from build123d import *

# Parameters (mm, degrees)
BOSS_EXTRU_1_DEPTH      = 10
ESQUISSE2_W             = 18.2
ESQUISSE2_H             = 8.4
ENL_V_MAT_EXTRU_1_DEPTH = 3
ESQUISSE3_R             = 1.6
ENL_V_MAT_EXTRU_2_DEPTH = 19.028865744
ESQUISSE4_R             = 3
ENL_V_MAT_EXTRU_3_DEPTH = 3
CONG_1_R                = 1.5


with BuildPart() as part:
    # Esquisse1 → Boss.-Extru.1 (new body)
    with BuildSketch(Plane(origin=(0, 0, 0), x_dir=(1, 0, 0), z_dir=(0, 1, 0))):
        Polygon((2.4, 0), (11, 0), (11, -9), (-11, -9), (-11, 0), (-2.4, 0), (-2.4, 1.2), (2.4, 1.2), align=None)
    extrude(amount=BOSS_EXTRU_1_DEPTH)

    # Esquisse2 → Enlèv. mat.-Extru.1 (cut)
    with BuildSketch(Plane(origin=(0, 10, 0), x_dir=(1, 0, 0), z_dir=(0, 1, 0))):
        with Locations((0, -3)):
            Rectangle(ESQUISSE2_W, ESQUISSE2_H)
    extrude(amount=-ENL_V_MAT_EXTRU_1_DEPTH, mode=Mode.SUBTRACT)

    # Esquisse3 → Enlèv. mat.-Extru.2 (cut, through all)
    with BuildSketch(Plane(origin=(0, 0, -1.2), x_dir=(-1, 0, 0), z_dir=(0, 0, -1))):
        with Locations((0, 3.5)):
            Circle(ESQUISSE3_R)
    extrude(amount=-ENL_V_MAT_EXTRU_2_DEPTH, mode=Mode.SUBTRACT)

    # Esquisse4 → Enlèv. mat.-Extru.3 (cut)
    with BuildSketch(Plane.XY.offset(9)):
        with Locations((0, 3.5)):
            Circle(ESQUISSE4_R)
    extrude(amount=-ENL_V_MAT_EXTRU_3_DEPTH, mode=Mode.SUBTRACT)

    # Congé1
    # the kernel refuses this fillet: 1.5 mm, written as the material it takes off along each edge
    with BuildSketch(Plane(origin=(9.5, 8.5, 7.5), x_dir=(0, 1, 0), z_dir=(1, 0, 0))) as cong_1_piece_1_section:
        Polygon((0, 0), (CONG_1_R, 0), (CONG_1_R, CONG_1_R), (0, CONG_1_R), align=None)
    cong_1_piece_1 = extrude(amount=CONG_1_R, mode=Mode.PRIVATE)
    cong_1_piece_1 = cong_1_piece_1 - Plane(origin=(9.5, 8.5, 7.5), x_dir=(0, -0.7071067811865475, -0.7071067811865475), z_dir=(1, 0, 0)) * Sphere(CONG_1_R, mode=Mode.PRIVATE)
    add(cong_1_piece_1, mode=Mode.SUBTRACT)
    with BuildSketch(Plane(origin=(9.5, 1.5, 7.5), x_dir=(1, 0, 0), z_dir=(0, -1, 0))) as cong_1_piece_2_section:
        Polygon((0, 0), (CONG_1_R, 0), (CONG_1_R, CONG_1_R), (0, CONG_1_R), align=None)
    cong_1_piece_2 = extrude(amount=CONG_1_R, mode=Mode.PRIVATE)
    cong_1_piece_2 = cong_1_piece_2 - Plane(origin=(9.5, 1.5, 7.5), x_dir=(-0.7071067811865476, 0, -0.7071067811865475), z_dir=(0, -1, 0)) * Sphere(CONG_1_R, mode=Mode.PRIVATE)
    add(cong_1_piece_2, mode=Mode.SUBTRACT)
    with BuildSketch(Plane(origin=(-9.5, 1.5, 7.5), x_dir=(0, -1, 0), z_dir=(-1, 0, 0))) as cong_1_piece_3_section:
        Polygon((0, 0), (CONG_1_R, 0), (CONG_1_R, CONG_1_R), (0, CONG_1_R), align=None)
    cong_1_piece_3 = extrude(amount=CONG_1_R, mode=Mode.PRIVATE)
    cong_1_piece_3 = cong_1_piece_3 - Plane(origin=(-9.5, 1.5, 7.5), x_dir=(0, 0.7071067811865475, -0.7071067811865475), z_dir=(-1, 0, 0)) * Sphere(CONG_1_R, mode=Mode.PRIVATE)
    add(cong_1_piece_3, mode=Mode.SUBTRACT)
    with BuildSketch(Plane(origin=(-9.5, 8.5, 7.5), x_dir=(0, 1, 0), z_dir=(-1, 0, 0))) as cong_1_piece_4_section:
        Polygon((0, 0), (CONG_1_R, 0), (CONG_1_R, -CONG_1_R), (0, -CONG_1_R), align=None)
    cong_1_piece_4 = extrude(amount=CONG_1_R, mode=Mode.PRIVATE)
    cong_1_piece_4 = cong_1_piece_4 - Plane(origin=(-9.5, 8.5, 7.5), x_dir=(0, -0.7071067811865475, -0.7071067811865475), z_dir=(-1, 0, 0)) * Sphere(CONG_1_R, mode=Mode.PRIVATE)
    add(cong_1_piece_4, mode=Mode.SUBTRACT)
    with BuildSketch(Plane(origin=(11, 10, -3.75), x_dir=(0, -1, 0), z_dir=(0, 0, 1)), Plane(origin=(-11, 0, 7.5), x_dir=(1, 0, 0), z_dir=(0, 0, -1)), Plane(origin=(11, 0, -3.75), x_dir=(-1, 0, 0), z_dir=(0, 0, 1))) as cong_1_piece_5:
        with BuildLine():
            CenterArc((CONG_1_R, -CONG_1_R), CONG_1_R, 90, 90)
            Line((0, -CONG_1_R), (0, 0))
            Line((0, 0), (CONG_1_R, 0))
        make_face()
    extrude(amount=11.25, mode=Mode.SUBTRACT)
    with BuildSketch(Plane(origin=(9.5, 0, 9), x_dir=(0, 0, -1), z_dir=(-1, 0, 0))) as cong_1_piece_6:
        with BuildLine():
            CenterArc((CONG_1_R, -CONG_1_R), CONG_1_R, 90, 90)
            Line((0, -CONG_1_R), (0, 0))
            Line((0, 0), (CONG_1_R, 0))
        make_face()
    extrude(amount=19, mode=Mode.SUBTRACT)
    with BuildSketch(Plane(origin=(-11, -3.75, 0), x_dir=(0, 0, 1), z_dir=(0, 1, 0)), Plane(origin=(11, -3.75, 0), x_dir=(-1, 0, 0), z_dir=(0, 1, 0))) as cong_1_piece_7:
        with BuildLine():
            CenterArc((CONG_1_R, CONG_1_R), CONG_1_R, 180, 90)
            Line((0, CONG_1_R), (0, 0))
            Line((0, 0), (CONG_1_R, 0))
        make_face()
    extrude(amount=17.5, mode=Mode.SUBTRACT)
    with BuildSketch(Plane(origin=(11, 1.5, 9), x_dir=(0, 0, -1), z_dir=(0, 1, 0)), Plane(origin=(-11, 1.5, 9), x_dir=(1, 0, 0), z_dir=(0, 1, 0))) as cong_1_piece_8:
        with BuildLine():
            CenterArc((CONG_1_R, CONG_1_R), CONG_1_R, 180, 90)
            Line((0, CONG_1_R), (0, 0))
            Line((0, 0), (CONG_1_R, 0))
        make_face()
    extrude(amount=7, mode=Mode.SUBTRACT)
    with BuildSketch(Plane(origin=(2.4, 7, 0), x_dir=(-1, 0, 0), z_dir=(0, 0, -1)), Plane(origin=(-2.4, 7, -4.95), x_dir=(1, 0, 0), z_dir=(0, 0, 1)), Plane(origin=(-2.4, 0, 0), x_dir=(1, 0, 0), z_dir=(0, 0, -1)), Plane(origin=(2.4, 0, -4.95), x_dir=(-1, 0, 0), z_dir=(0, 0, 1))) as cong_1_piece_9:
        with BuildLine():
            CenterArc((CONG_1_R, -CONG_1_R), CONG_1_R, 90, 90)
            Line((0, -CONG_1_R), (0, 0))
            Line((0, 0), (CONG_1_R, 0))
        make_face()
    extrude(amount=4.95, mode=Mode.SUBTRACT)
    with BuildSketch(Plane(origin=(-11, 10, 7.5), x_dir=(1, 0, 0), z_dir=(0, 0, -1))) as cong_1_piece_10:
        with BuildLine():
            CenterArc((CONG_1_R, CONG_1_R), CONG_1_R, 180, 90)
            Line((0, CONG_1_R), (0, 0))
            Line((0, 0), (CONG_1_R, 0))
        make_face()
    extrude(amount=11.25, mode=Mode.SUBTRACT)
    with BuildSketch(Plane(origin=(9.5, 10, 9), x_dir=(0, 0, -1), z_dir=(-1, 0, 0))) as cong_1_piece_11:
        with BuildLine():
            CenterArc((CONG_1_R, CONG_1_R), CONG_1_R, 180, 90)
            Line((0, CONG_1_R), (0, 0))
            Line((0, 0), (CONG_1_R, 0))
        make_face()
    extrude(amount=19, mode=Mode.SUBTRACT)


solid = part.part
Geometry check sheet. Reference: the model listing, model coordinates, mm. A direction names the side the tool comes from. Give positions to 0.01 mm unless a question says otherwise; leave off trailing zeros. Order: outer loops, then holes, each group sorted by start corner. A loop starts at its lowest first (then second) coordinate and runs counter-clockwise, first axis right, second up.
1) Cross-section at B-B (z = 4.25). Record the boundary of the cut face in (x, y).
Results are:
outline: (-11, 1.5) arc R1.5 ccw to (-9.5, 0) - (9.5, 0) arc R1.5 ccw to (11, 1.5) - (11, 8.5) arc R1.5 ccw to (9.5, 10) - (9.1, 10) - (9.1, 7) - (-9.1, 7) - (-9.1, 10) - (-9.5, 10) arc R1.5 ccw to (-11, 8.5) - close; hole circle Ø3.2 at (0, 3.5)
2) Draft check along Y on faces 1 (the cylindrical face through (-10.55, 0.43, 3.8)), 2 (the flat face through (11, 5, 4)), 3 (the cylindrical face through (1.95, 6.57, -0.59)), 4 (the flat face through (1, 2, 6)). Enter one of: released by +Y, released by -Y, zero draft, split by the parting line, or undercut.
Results are:
face 1: released by -Y
face 2: zero draft
face 3: released by +Y
face 4: undercut
3) Tool access check on faces 5 (the flat face through (0, 9, 7.2)), 6 (the flat face through (2.4, 3, -1)), 7 (the cylindrical face through (-1.95, 0.43, -0.59)), 8 (the cylindrical face through (-0.391, 6.474, 7.521)), 9 (the flat face through (-2.4, 3, -1)). Record the directions out of +Z, -Z, +X, -X, +Y, -Y that give a thin tool (end or side, any length) a straight path to the whole face; none if there is none.
Results are:
face 5: -Z, +Y
face 6: -Z, +X, +Y, -Y
face 7: -Z, -X, -Y
face 8: +Z
face 9: -Z, -X, +Y, -Y
4) Cross-section at A-A (y = 3.5). Record the boundary of the cut face in (x, z), then the cut area to 3 significant figures.
Results are:
outline: (-11, 1.5) arc R1.5 ccw to (-9.5, 0) - (-2.4, 0) - (-2.4, -1.2) - (-1.6, -1.2) - (-1.6, 6) - (-3, 6) - (-3, 9) - (-9.5, 9) arc R1.5 ccw to (-11, 7.5) - close; (1.6, -1.2) - (2.4, -1.2) - (2.4, 0) - (9.5, 0) arc R1.5 ccw to (11, 1.5) - (11, 7.5) arc R1.5 ccw to (9.5, 9) - (3, 9) - (3, 6) - (1.6, 6) - close
area: 161 mm2
5) Cross-section at C-C (x = 0). Record the boundary of the cut face in (y, z), then the cut area to 3 significant figures.
Results are:
outline: (0, -1.2) - (1.9, -1.2) - (1.9, 6) - (0.5, 6) - (0.5, 8.62) arc R1.5 ccw to (0, 7.5) - close; (5.1, -1.2) - (7, -1.2) - (7, 7.2) - (10, 7.2) - (10, 7.5) arc R1.5 ccw to (8.5, 9) - (6.5, 9) - (6.5, 6) - (5.1, 6) - close
area: 34.9 mm2
6) Material ranges on probe 1 along X at (y, z) = (3.5, 7.1); probe 2 along Y at (x, z) = (0, 7.6); probe 3 along Y at (x, z) = (0, 3.75), recorded low to high.
Results are:
probe 1: x = -11 to -3, 3 to 11
probe 2: y = 0 to 0.5, 6.5 to 10
probe 3: y = 0 to 1.9, 5.1 to 7
7) Cross-section at D-D (x = 7.75). Record the boundary of the cut face in (y, z), then the cut area to 3 significant figures.
Results are:
outline: (0, 0) - (7, 0) - (7, 7.2) - (10, 7.2) - (10, 7.5) arc R1.5 ccw to (8.5, 9) - (1.5, 9) arc R1.5 ccw to (0, 7.5) - close
area: 67.4 mm2
8) Gauge pin test, flat ends, axial feed: pin 1 (1.5 mm diameter, centred on x = -2, y = 8, fed in from -Z); pin 2 (3 mm diameter, centred on x = -0.5, z = 0, fed in from -Y); pin 3 (3.5 mm diameter, centred on x = 0, y = 3.5, fed in from +Z); pin 4 (1 mm diameter, centred on x = 4, z = 0.5, fed in from +Y). Record the tip position at first contact, or that the pin passes through.
Results are:
pin 1: stops at z = 7.2
pin 2: stops at y = 0
pin 3: stops at z = 6
pin 4: stops at y = 7
